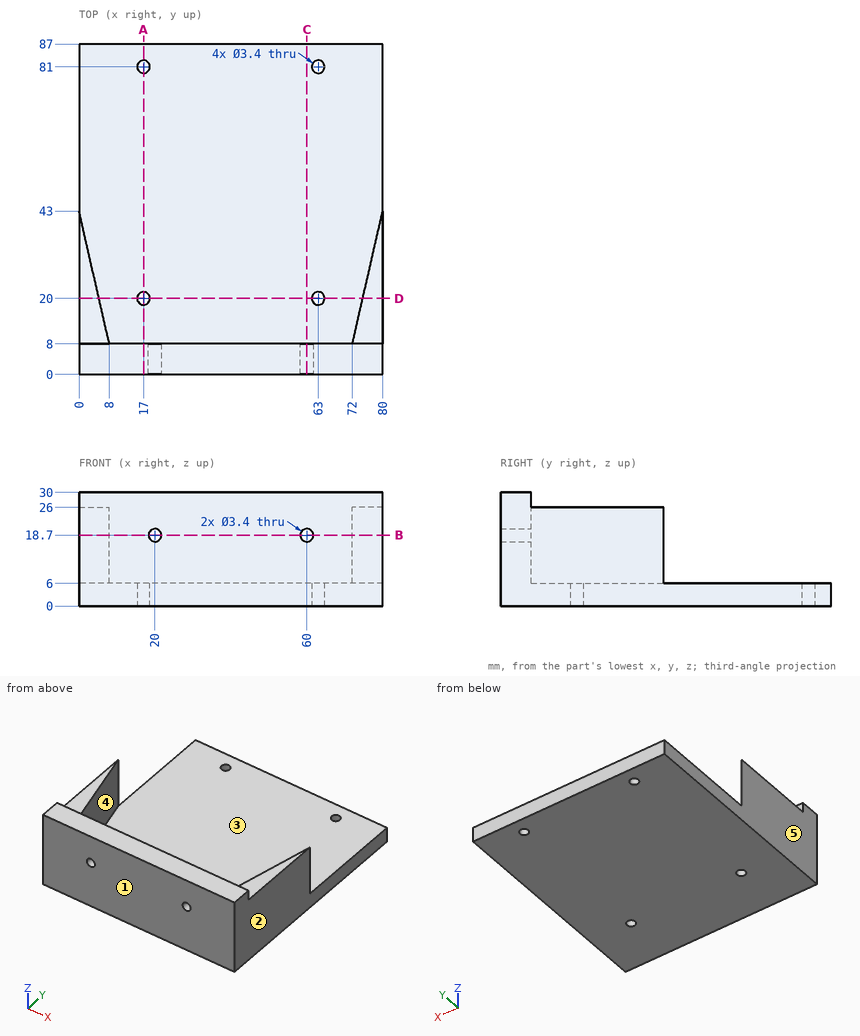
The drawing under review shows one solid part. Ordinate dimensions are in mm from its lowest x, y, z. A direction names the side the tool comes from. Coordinates: 2 decimals unless noted, no trailing zeros. Write each loop counter-clockwise with the first axis right and the second up, starting at its lowest first coordinate (ties: lowest second). Pieces come first, ordered by that corner, then holes. Notation, with made-up numbers: (69.25, -8.5) - (105.25, -8.5) arc R33 cw to (105.25, 22.5) - close; hole circle Ø10 at (23, 88). An arc over 180 degrees is marked (long way). Answer in a Markdown table with one row per item. Add a question column.
Q1. For probe 1 along X at (y, z) = (81, 3.1); probe 2 along Y at (x, z) = (17, 2); probe 3 along Y at (x, z) = (36, 22.75), list the stretches that pass through material, from the lowest coordinate up.
Q2. We need section B-B, the plane z = 18.7. State the section outline as (x, y) points, and give its area (3 significant figures).
Q3. Draft analysis for pull direction X (two halves, no side actions). For the marked faces 1, 2 and 3, state which applies: +X half, -X half, draft (parallel to the pull), parting line (faces both ways), or undercut.
Q4. Tool access review of the marked faces 4 and 5: name each direction out of +Z, -Z, +X, -X, +Y, -Y from which nothing blocks a thin tool from reaching the whole face with its end or side.
Q5. We need section A-A, the plane x = 17. State the section outline as (y, z) points.
Q6. We need section C-C, the plane x = 60. State the section outline as (y, z) points.
Q7. For P1, Ø5.5, axis at x = 17, y = 20, coming from the -Z side; P2, Ø6.5, axis at x = 75, y = 34, coming from the +Z side; P3, Ø1, axis at x = 28.5, z = 16, coming from the +Y side; P4, Ø23.5, axis at x = 56.5, y = 56.5, coming from the +Z side, all flat-tipped, find the tip position at first contact; note any pin that passes through.
Q8. We need section D-D, the plane y = 20. State the section outline as (x, z) points.
Answer list:
| question | item | result |
|---|---|---|
| 1 | probe 1 | x = 0 to 15.3, 18.7 to 61.3, 64.7 to 80 |
| 1 | probe 2 | y = 0 to 18.3, 21.7 to 79.3, 82.7 to 87 |
| 1 | probe 3 | y = 0 to 8 |
| 2 | outline | (0, 0) - (18.3, 0) - (18.3, 8) - (8, 8) - (0, 43) - close; (21.7, 0) - (58.3, 0) - (58.3, 8) - (21.7, 8) - close; (61.7, 0) - (80, 0) - (80, 43) - (72, 8) - (61.7, 8) - close |
| 2 | area | 866 mm2 |
| 3 | face 1 | draft |
| 3 | face 2 | +X half |
| 3 | face 3 | undercut |
| 4 | face 4 | +Z, +Y |
| 4 | face 5 | +Z, -Z, -X, +Y, -Y |
| 5 | outline | (0, 0) - (18.3, 0) - (18.3, 6) - (8, 6) - (8, 30) - (0, 30) - close; (21.7, 0) - (79.3, 0) - (79.3, 6) - (21.7, 6) - close; (82.7, 0) - (87, 0) - (87, 6) - (82.7, 6) - close |
| 6 | outline | (0, 0) - (87, 0) - (87, 6) - (8, 6) - (8, 17) - (0, 17) - close; (0, 20.4) - (8, 20.4) - (8, 30) - (0, 30) - close |
| 7 | P1 | stops at z = 0 |
| 7 | P2 | stops at z = 26 |
| 7 | P3 | stops at y = 8 |
| 7 | P4 | stops at z = 6 |
| 8 | outline | (0, 0) - (15.3, 0) - (15.3, 6) - (5.26, 6) - (5.26, 26) - (0, 26) - close; (18.7, 0) - (61.3, 0) - (61.3, 6) - (18.7, 6) - close; (64.7, 0) - (80, 0) - (80, 26) - (74.74, 26) - (74.74, 6) - (64.7, 6) - close |
